Source: CAD feature listing. Evaluate the final solid. Frame: model axes, mm. Round coordinates to 2 decimals unless told otherwise and drop trailing zeros. Order: outer loops, then holes, each group sorted by start corner. A loop starts at its lowest first (then second) coordinate and runs counter-clockwise, first axis right, second up. Notation, with made-up numbers: (-26, -27) -> (25, -27) arc R24 ccw to (25, 6) -> close; hole circle Ø5 at (5.5, 17.5). An arc over 180 degrees is marked (long way). Answer as CSV lines item,"result". Start each with the question number.
(1) Section query B-B (x = 0). Output: boundary loops of the cut face in (y, z).
(2) Line query: line 1 along Y through (x, z) = (-0.5, 1.5); line 2 along Y through (x, z) = (-2, 0.75). Output: solid intervals per line, ascending. Write a range as from..to.
(3) Section query A-A (z = 1.2). Output: boundary loops of the cut face in (x, y), plus the area to 3 significant figures.
```python
from build123d import *

# Parameters (mm, degrees)
SKETCH1_W           = 60
SKETCH1_H           = 634.64
BOSS_EXTRUDE1_DEPTH = 2
CUT_EXTRUDE1_REACH  = 320.741


with BuildPart() as part:
    # Sketch1 → Boss-Extrude1 (new body)
    with BuildSketch(Plane.XY):
        Rectangle(SKETCH1_W, SKETCH1_H)
    extrude(amount=BOSS_EXTRUDE1_DEPTH)

    # Sketch2 → Cut-Extrude1 (cut, up to next)
    with BuildSketch(Plane.XY.offset(2), mode=Mode.PRIVATE) as cut_extrude1_sk1:
        with BuildLine():
            Line((7.5, 294.82), (7.5, 279.82))
            ThreePointArc((7.5, 279.82), (0, 272.32), (-7.5, 279.82))
            Line((-7.5, 279.82), (-7.5, 294.82))
            ThreePointArc((-7.5, 294.82), (0, 302.32), (7.5, 294.82))
        make_face()
    cut_extrude1_tool1 = extrude(cut_extrude1_sk1.sketch, amount=-CUT_EXTRUDE1_REACH, mode=Mode.PRIVATE) & part.part
    # Sketch2 → Cut-Extrude1 (cut, up to next)
    with BuildSketch(Plane.XY.offset(2), mode=Mode.PRIVATE) as cut_extrude1_sk2:
        with BuildLine():
            Line((7.5, -294.82), (7.5, -279.82))
            ThreePointArc((7.5, -279.82), (0, -272.32), (-7.5, -279.82))
            Line((-7.5, -279.82), (-7.5, -294.82))
            ThreePointArc((-7.5, -294.82), (0, -302.32), (7.5, -294.82))
        make_face()
    cut_extrude1_tool2 = extrude(cut_extrude1_sk2.sketch, amount=-CUT_EXTRUDE1_REACH, mode=Mode.PRIVATE) & part.part
    add(cut_extrude1_tool1.solids().sort_by_distance((0, 287.32, 2))[0], mode=Mode.SUBTRACT)
    add(cut_extrude1_tool2.solids().sort_by_distance((0, -287.32, 2))[0], mode=Mode.SUBTRACT)


solid = part.part
```
Answer block:
1,outline,"(-317.32, 0) -> (-302.32, 0) -> (-302.32, 2) -> (-317.32, 2) -> close; (-272.32, 0) -> (272.32, 0) -> (272.32, 2) -> (-272.32, 2) -> close; (302.32, 0) -> (317.32, 0) -> (317.32, 2) -> (302.32, 2) -> close"
2,line 1,"-317.32..-302.3, -272.34..272.34, 302.3..317.32"
2,line 2,"-317.32..-302.05, -272.59..272.59, 302.05..317.32"
3,outline,"(-30, -317.32) -> (30, -317.32) -> (30, 317.32) -> (-30, 317.32) -> close; hole (-7.5, -294.82) arc R7.5 ccw to (7.5, -294.82) -> (7.5, -279.82) arc R7.5 ccw to (-7.5, -279.82) -> close; hole (-7.5, 279.82) arc R7.5 ccw to (7.5, 279.82) -> (7.5, 294.82) arc R7.5 ccw to (-7.5, 294.82) -> close"
3,area,"37,300 mm2"
